Geometry check sheet. Reference: drawing and pictorial views, mm from the part's lowest x, y, z. Give positions to 0.01 mm unless a question says otherwise; leave off trailing zeros. Write each loop counter-clockwise with the first axis right and the second up, starting at its lowest first coordinate (ties: lowest second). Pieces come first, ordered by that corner, then holes. Notation, with made-up numbers: M 16.5,60 L 65.5,60 A32 ccw 65.5,95 Z; hole C 14,-5.75 d6. An arc over 180 degrees is marked long. One line per item, written item: value. Start each with the question number.
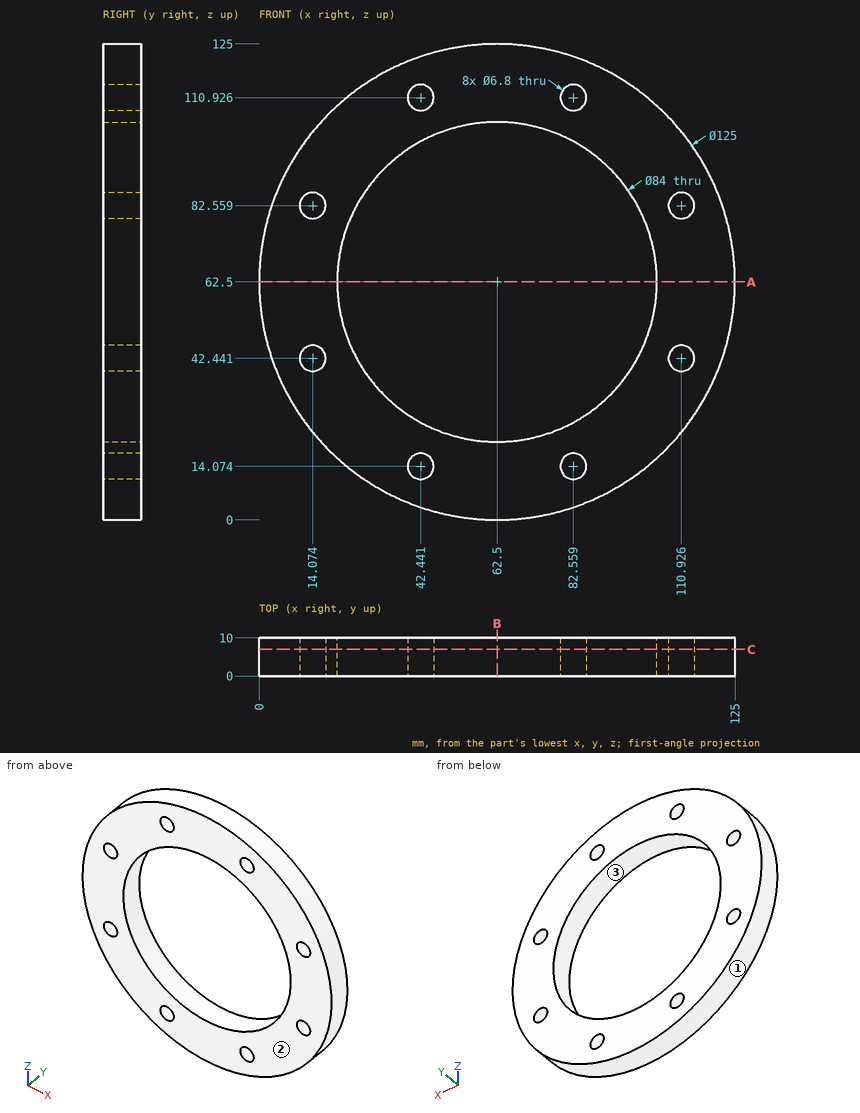
1) Cross-section at B-B (x = 62.5). Record the boundary of the cut face in (y, z), plus the area to 3 significant figures.
2) Gauge pin test, flat ends, axial feed: pin 1 (6 mm diameter, centred on x = 43.5, y = 7, fed in from +Z); pin 2 (1 mm diameter, centred on y = 4.5, z = 36.5, fed in from -X); pin 3 (3 mm diameter, centred on x = 30.5, y = 6.5, fed in from +Z). Record the tip position at first contact, or that the pin passes through.
3) Material ranges on L1, parallel to Z at x = 63, y = 5.5; L2, parallel to X at y = 1, z = 84 (1 decimal); L3, parallel to Z at x = 39.5, y = 4 (1 decimal), recorded low to high. Write a range as from..to.
4) Cross-section at A-A (z = 62.5). Record the boundary of the cut face in (x, y).
5) Cross-section at C-C (y = 7). State how many separate pieces and enclosed holes the cut face has, plus the area to 3 significant figures.
6) Draft check along Z on the marked faces 1, 2 and 3. Enter one of: released by +Z, released by -Z, zero draft, split by the parting line, or undercut.
Data:
1. outline: M 0,0 L 10,0 L 10,20.5 L 0,20.5 Z; M 0,104.5 L 10,104.5 L 10,125 L 0,125 Z
1. area: 410 mm2
2. pin 1: stops at z = 122.92
2. pin 2: stops at x = 5.44
2. pin 3: stops at z = 117.05
3. L1: z = 0..20.5, 104.5..125
3. L2: x = 3.8..11, 17.2..26.4, 98.6..107.8, 114..121.2
3. L3: z = 4.4..12.4, 15.8..27.4, 97.6..109.2, 112.6..120.6
4. outline: M 0,0 L 20.5,0 L 20.5,10 L 0,10 Z; M 104.5,0 L 125,0 L 125,10 L 104.5,10 Z
5. separate pieces: 1
5. enclosed holes: 9
5. area: 6,440 mm2
6. face 1: split by the parting line
6. face 2: zero draft
6. face 3: undercut
